For this review, take the finished solid that the model builds, in its own axes (mm). Coordinates: 2 decimals unless noted, no trailing zeros. Loops run counter-clockwise (first coordinate to the right, second up) from the corner with the lowest first, then second, coordinate; pieces in that order, holes last. Notation, with made-up numbers: M 39,-26 L 90,-26 A26 cw 90,11 Z; hole C 84.25,-26 d1. An arc over 180 degrees is marked long. Use one line per item in the form item = value.
```python
from build123d import *

# Parameters (mm, degrees)
RESSALTO_EXTRUS_O2_DEPTH = 10
ESBO_O3_R                = 1
ESBO_O3_R_2              = 3
CORTE_EXTRUS_O1_DEPTH    = 87.670292346


with BuildPart() as part:
    # Esboço2 → Ressalto-extrusão2 (new body)
    with BuildSketch(Plane(origin=(0, 0, 0), x_dir=(0, 0, -1), z_dir=(1, 0, 0))):
        Polygon((69.5, -29.489859634), (77.5, -29.489859634), (77.5, -37.489859634), (-76.5, -37.489859634), (-76.5, -29.489859634), (-68.5, -29.489859634), (-68.5, -3.948025217), (-4.978169529, 1.609414836), (0, 1.609414836), (5.978169529, 1.609414836), (69.5, -3.948025217), align=None)
    extrude(amount=RESSALTO_EXTRUS_O2_DEPTH)

    # Esboço3 → Corte-extrusão1 (cut, through all)
    with BuildSketch(Plane(origin=(10, 0, 0), x_dir=(0, 0, -1), z_dir=(1, 0, 0))):
        with Locations((0.5, -8.390585169)):
            Circle(ESBO_O3_R)
        with Locations((0.5, -27.002843355)):
            Circle(ESBO_O3_R_2)
        with Locations((57.5, -13.178770401)):
            Circle(ESBO_O3_R_2)
        with Locations((57.5, -29.489859634)):
            Circle(ESBO_O3_R)
        with Locations((-56.5, -13.178770401)):
            Circle(ESBO_O3_R_2)
        with Locations((-56.5, -29.489859634)):
            Circle(ESBO_O3_R)
    extrude(amount=-CORTE_EXTRUS_O1_DEPTH, mode=Mode.SUBTRACT)


solid = part.part
```
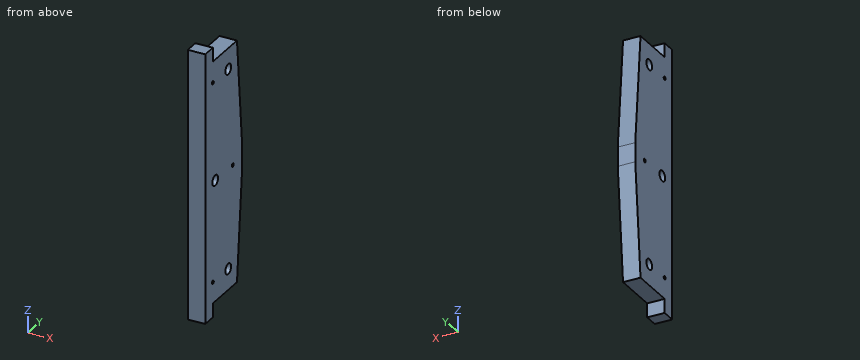
1. Consider section C-C on z = -33. Write out the cut boundary in (x, y), plus the area to 3 significant figures.
Computed values:
outline = M 0,-37.49 L 10,-37.49 L 10,-0.75 L 0,-0.75 Z
area = 367 mm2
2. Consider section A-A on x = 4. Write out the cut boundary in (y, z).
Computed values:
outline = M -37.49,-77.5 L -29.49,-77.5 L -29.49,-69.5 L -3.95,-69.5 L 1.61,-5.98 L 1.61,4.98 L -3.95,68.5 L -29.49,68.5 L -29.49,76.5 L -37.49,76.5 Z; hole C -29.49,-57.5 d2; hole C -29.49,56.5 d2; hole C -27,-0.5 d6; hole C -13.18,-57.5 d6; hole C -13.18,56.5 d6; hole C -8.39,-0.5 d2
3. Consider section B-B on z = 64.5. Write out the cut boundary in (x, y), plus the area to 3 significant figures.
Computed values:
outline = M 0,-37.49 L 10,-37.49 L 10,-3.6 L 0,-3.6 Z
area = 339 mm2
4. Wall thickness on line 1 along Z through (x, y) = (0.5, -10.5); line 2 along Z through (x, y) = (2.25, -14.5); line 3 along Y through (x, z) = (7, 56): over which ranges is each line inside the solid? List them lowest first. Write a range as from..to.
Computed values:
line_1 = -69.5..-58.85, -56.15..55.15, 57.85..68.5
line_2 = -69.5..-60.19, -54.81..53.81, 59.19..68.5
line_3 = -37.49..-30.36, -28.62..-16.14, -10.22..-2.85
5. For pin 1 Ø4 at (x, z) = (7.5, -73) entering from +Y; pin 2 Ø1.2 at (y, z) = (-8.39, -0.5) entering from -X; pin 3 Ø3 at (x, z) = (2.5, -56) entering from +Y; pin 4 Ø5 at (x, y) = (5.5, -18.5) entering from -Z, all flat-tipped, find the tip position at first contact; note any pin that passes through.
Computed values:
pin_1 = -29.49
pin_2 = through
pin_3 = -2.64
pin_4 = -69.5
